Autodesk Inventor part; units mm, degrees
ref_plane "YZ Plane" through (0, 0, 0) normal (1, 0, 0) x (0, 1, 0)
ref_plane "XZ Plane" through (0, 0, 0) normal (0, 1, 0) x (-1, 0, 0)
ref_plane "XY Plane" through (0, 0, 0) normal (0, 0, 1) x (1, 0, 0)
sketch "Sombreado_1" plane through (0, 0, 0) normal (0, 0, 1) x (1, 0, 0)
  point P0 (0, 0)
sketch "Sombreado_2" plane through (0, 0, 0) normal (0, 0, 1) x (1, 0, 0)
  point P0 (0, 0)
sketch "Sombreado_3" plane through (0, 0, 0) normal (0, 0, 1) x (1, 0, 0)
  point P0 (0, 0)
sketch "Boceto1" plane through (0, 0, 0) normal (0, 1, 0) x (-1, 0, 0)
  line L0 (30.3882, 1.25) -> (30.8882, 1.25)
  line L1 (0, -6.75) -> (75, -6.75)
  line L2 (75, -6.75) -> (75, 18.25)
  line L3 (75, 18.25) -> (0, 18.25)
  line L4 (0, 18.25) -> (0, -6.75)
  arc A0 (21.3882, 1.25) -> (30.8882, 1.25) centre (26.1382, 1.25) ccw
  arc A1 (21.8882, 1.25) -> (30.3882, 1.25) centre (26.1382, 1.25) ccw
  line L5 (21.3882, 1.25) -> (21.8882, 1.25)
  line L6 (1.8, 2.5) -> (5.3, 2.5)
  line L7 (1.8, 2.5) -> (1.8, 3)
  line L8 (1.8, 3) -> (1, 3)
  line L9 (1, 3) -> (1, 2.5)
  line L10 (1, 0) -> (0, 0)
  line L11 (1, 0) -> (1, -0.5)
  line L12 (1, -0.5) -> (1.8, -0.5)
  line L13 (1.8, -0.5) -> (1.8, 0)
  line L14 (5.3, 0) -> (1.8, 0)
  line L15 (0, 2.5) -> (1, 2.5)
  line L16 (1.8, 11.5) -> (5.3, 11.5)
  line L17 (5.3, 9) -> (1.8, 9)
  line L18 (1, 9) -> (0, 9)
  line L19 (0, 11.5) -> (1, 11.5)
  line L20 (1.8, 11.5) -> (1.8, 12)
  line L21 (1.8, 12) -> (1, 12)
  line L22 (1, 12) -> (1, 11.5)
  line L23 (1, 9) -> (1, 8.5)
  line L24 (1, 8.5) -> (1.8, 8.5)
  line L25 (1.8, 8.5) -> (1.8, 9)
  line L26 (44.6082, 1.25) -> (44.1082, 1.25)
  arc A2 (44.1082, 1.25) -> (53.6082, 1.25) centre (48.8582, 1.25) ccw
  arc A3 (44.6082, 1.25) -> (53.1082, 1.25) centre (48.8582, 1.25) ccw
  line L27 (53.6082, 1.25) -> (53.1082, 1.25)
  line L28 (73.1964, 2.5) -> (69.6964, 2.5)
  line L29 (69.6964, 0) -> (73.1964, 0)
  line L30 (73.9964, 0) -> (74.9964, 0)
  line L31 (74.9964, 2.5) -> (73.9964, 2.5)
  line L32 (73.1964, 2.5) -> (73.1964, 3)
  line L33 (73.1964, 3) -> (73.9964, 3)
  line L34 (73.9964, 3) -> (73.9964, 2.5)
  line L35 (73.9964, 0) -> (73.9964, -0.5)
  line L36 (73.9964, -0.5) -> (73.1964, -0.5)
  line L37 (73.1964, -0.5) -> (73.1964, 0)
  line L38 (73.1964, 11.5) -> (69.6964, 11.5)
  line L39 (69.6964, 9) -> (73.1964, 9)
  line L40 (73.9964, 9) -> (74.9964, 9)
  line L41 (74.9964, 11.5) -> (73.9964, 11.5)
  line L42 (73.1964, 11.5) -> (73.1964, 12)
  line L43 (73.1964, 12) -> (73.9964, 12)
  line L44 (73.9964, 12) -> (73.9964, 11.5)
  line L45 (73.9964, 9) -> (73.9964, 8.5)
  line L46 (73.9964, 8.5) -> (73.1964, 8.5)
  line L47 (73.1964, 8.5) -> (73.1964, 9)
  line L48 (75, 18.25) -> (75, 43.25)
  line L49 (75, 43.25) -> (0, 43.25)
  line L50 (0, 43.25) -> (0, 18.25)
  line L51 (5.3, 11.5) -> (5.3, 9)
  line L52 (5.3, 2.5) -> (5.3, 0)
  line L53 (69.6964, 11.5) -> (69.6964, 9)
  line L54 (69.6964, 2.5) -> (69.6964, 0)
  circle A4 centre (26.1382, 1.25) radius 3.25
  circle A5 centre (48.8582, 1.25) radius 3.25
  circle A6 centre (26.1382, 26.25) radius 3.25
  circle A7 centre (48.8582, 26.25) radius 3.25
  line L55 (75, 43.25) -> (75, 68.25)
  line L56 (75, 68.25) -> (0, 68.25)
  line L57 (0, 68.25) -> (0, 43.25)
  circle A8 centre (26.1382, 51.25) radius 3.25
  circle A9 centre (48.8582, 51.25) radius 3.25
  point P0 (0, 0)
sketch "Boceto3" plane through (0, 0, 0) normal (0, 1, 0) x (-1, 0, 0)
  line L0 (0, 0) -> (-75, 0)
  line L1 (-75, 0) -> (-75, -25)
  line L2 (-75, -25) -> (0, -25)
  line L3 (0, -25) -> (0, 0)
  line L4 (0, 0) -> (-75, 0)
  line L5 (-75, 0) -> (-75, -25)
  line L6 (-75, -25) -> (0, -25)
  line L7 (0, -25) -> (0, 0)
  dimension "d4" = 75
  dimension "d5" = 25
  dimension "d6" = 75
  dimension "d7" = 25
extrude "Extrusión1" add sketch "Boceto3" along normal blind 2
sketch "Boceto4" plane through (0, 2, 0) normal (0, 1, 0) x (1, 0, 0)
  line L0 (-1.8065, 18.25) -> (1.0036, 18.25)
  line L1 (-1.8065, 15.75) -> (1.0036, 15.75)
  line L2 (1.0036, 15.75) -> (1.0036, 15.25)
  line L3 (1.8036, 15.75) -> (1.8036, 15.25)
  line L4 (1.0036, 18.75) -> (1.8036, 18.75)
  line L5 (1.0036, 15.25) -> (1.8036, 15.25)
  line L6 (1.0036, 18.25) -> (1.0036, 18.75)
  line L7 (1.8036, 18.75) -> (1.8036, 18.25)
  line L8 (1.8036, 18.25) -> (5.3036, 18.25)
  line L9 (1.8036, 15.75) -> (5.3036, 15.75)
  line L10 (5.3036, 18.25) -> (5.3036, 15.75)
  line L11 (-1.5403, 9.25) -> (-1.5403, 6.75)
  line L12 (-1.5403, 9.25) -> (1.0036, 9.25)
  line L13 (-1.5403, 6.75) -> (1.0036, 6.75)
  line L14 (1.0036, 6.75) -> (1.0036, 6.25)
  line L15 (1.8036, 6.75) -> (1.8036, 6.25)
  line L16 (1.0036, 9.75) -> (1.8036, 9.75)
  line L17 (1.0036, 6.25) -> (1.8036, 6.25)
  line L18 (1.0036, 9.25) -> (1.0036, 9.75)
  line L19 (1.8036, 9.75) -> (1.8036, 9.25)
  line L20 (1.8036, 9.25) -> (5.3036, 9.25)
  line L21 (1.8036, 6.75) -> (5.3036, 6.75)
  line L22 (5.3036, 9.25) -> (5.3036, 6.75)
  circle A0 centre (26.1418, 8) radius 3.25
  arc A1 (21.3918, 8) -> (30.8918, 8) centre (26.1418, 8) ccw
  arc A2 (21.8918, 8) -> (30.3918, 8) centre (26.1418, 8) ccw
  line L23 (30.3918, 8) -> (30.8918, 8)
  line L24 (21.8918, 8) -> (21.3918, 8)
  line L25 (-1.8065, 18.25) -> (-1.8065, 15.75)
  line L26 (5.3036, 15.75) -> (7.3036, 16.75)
  line L27 (5.3036, 18.25) -> (7.3036, 17.25)
  line L28 (7.3036, 16.75) -> (9.4436, 16.75)
  line L29 (9.4436, 16.75) -> (13.6836, 12.5)
  line L30 (9.7963, 17.1027) -> (9.7972, 17.1036)
  line L31 (14.1397, 12.749) -> (9.6494, 17.25)
  line L32 (7.3036, 17.25) -> (9.6494, 17.25)
  line L33 (5.3036, 9.25) -> (7.3036, 8.25)
  line L34 (5.3036, 6.75) -> (7.3036, 7.75)
  line L35 (7.3036, 8.25) -> (9.4436, 8.25)
  line L36 (9.4436, 8.25) -> (13.6836, 12.5)
  line L37 (14.1397, 12.251) -> (9.6494, 7.75)
  line L38 (7.3036, 7.75) -> (9.6494, 7.75)
  line L39 (14.1397, 12.749) -> (26.1418, 12.749)
  line L40 (14.1397, 12.251) -> (26.1418, 12.251)
  arc A3 (30.3918, 8) -> (26.1418, 12.25) centre (26.1418, 8) ccw
  arc A4 (30.8918, 8) -> (26.1418, 12.75) centre (26.1418, 8) ccw
  line L41 (0, 0) -> (75, 0)
  line L42 (75, 25) -> (0, 25)
  line L43 (76.8065, 18.25) -> (73.9964, 18.25)
  line L44 (76.8065, 15.75) -> (73.9964, 15.75)
  line L45 (73.9964, 15.75) -> (73.9964, 15.25)
  line L46 (73.1964, 15.75) -> (73.1964, 15.25)
  line L47 (73.9964, 18.75) -> (73.1964, 18.75)
  line L48 (73.9964, 15.25) -> (73.1964, 15.25)
  line L49 (73.9964, 18.25) -> (73.9964, 18.75)
  line L50 (73.1964, 18.75) -> (73.1964, 18.25)
  line L51 (73.1964, 18.25) -> (69.6964, 18.25)
  line L52 (73.1964, 15.75) -> (69.6964, 15.75)
  line L53 (69.6964, 18.25) -> (69.6964, 15.75)
  line L54 (69.6964, 9.25) -> (69.6964, 6.75)
  line L55 (73.1964, 6.75) -> (73.1964, 6.25)
  line L56 (73.1964, 6.75) -> (69.6964, 6.75)
  line L57 (73.1964, 9.75) -> (73.1964, 9.25)
  line L58 (73.9964, 6.75) -> (73.9964, 6.25)
  line L59 (73.9964, 6.25) -> (73.1964, 6.25)
  line L60 (73.9964, 9.75) -> (73.1964, 9.75)
  line L61 (73.9964, 9.25) -> (73.9964, 9.75)
  line L62 (76.5403, 9.25) -> (76.5403, 6.75)
  line L63 (76.5403, 9.25) -> (73.9964, 9.25)
  line L64 (76.5403, 6.75) -> (73.9964, 6.75)
  line L65 (73.1964, 9.25) -> (69.6964, 9.25)
  circle A5 centre (48.8582, 8) radius 3.25
  arc A6 (44.1082, 8) -> (53.6082, 8) centre (48.8582, 8) ccw
  arc A7 (44.6082, 8) -> (53.1082, 8) centre (48.8582, 8) ccw
  line L66 (44.6082, 8) -> (44.1082, 8)
  line L67 (53.1082, 8) -> (53.6082, 8)
  line L68 (76.8065, 18.25) -> (76.8065, 15.75)
  line L69 (69.6964, 15.75) -> (67.6964, 16.75)
  line L70 (69.6964, 18.25) -> (67.6964, 17.25)
  line L71 (67.6964, 16.75) -> (65.5564, 16.75)
  line L72 (65.5564, 16.75) -> (61.3164, 12.5)
  line L73 (65.2037, 17.1027) -> (65.2028, 17.1036)
  line L74 (60.8603, 12.749) -> (65.3506, 17.25)
  line L75 (67.6964, 17.25) -> (65.3506, 17.25)
  line L76 (67.6964, 8.25) -> (65.5564, 8.25)
  line L77 (67.6964, 7.75) -> (65.3506, 7.75)
  line L78 (60.8603, 12.251) -> (65.3506, 7.75)
  line L79 (65.5564, 8.25) -> (61.3164, 12.5)
  line L80 (69.6964, 9.25) -> (67.6964, 8.25)
  line L81 (69.6964, 6.75) -> (67.6964, 7.75)
  line L82 (60.8603, 12.749) -> (48.8582, 12.749)
  line L83 (60.8603, 12.251) -> (48.8582, 12.251)
  arc A8 (48.8582, 12.25) -> (44.6082, 8) centre (48.8582, 8) ccw
  arc A9 (48.8582, 12.75) -> (44.1082, 8) centre (48.8582, 8) ccw
extrude "Extrusión2" cut sketch "Boceto4" against normal blind 2 contours L0 L6 L4 L7 L8 L10 L9 L3 L5 L2 L1 L25 | A1 L24 A2 L23 | L22 L21 L15 L17 L14 L13 L11 L12 L18 L16 L19 L20 | A0 | L68 L44 L45 L48 L46 L52 L53 L51 L50 L47 L49 L43 | L66 A7 L67 A6 | L65 L57 L60 L61 L63 L62 L64 L58 L59 L55 L56 L54 | A5
sketch "Boceto5" plane through (0, 2, 0) normal (0, 1, 0) x (1, 0, 0)
  line L0 (5.3036, 18.25) -> (5.3036, 15.75)
  line L1 (5.3036, 9.25) -> (5.3036, 6.75)
  line L2 (5.3036, 15.75) -> (7.3036, 16.75)
  line L3 (5.3036, 18.25) -> (7.3036, 17.25)
  line L4 (7.3036, 16.75) -> (9.4436, 16.75)
  line L5 (9.4436, 16.75) -> (13.6836, 12.5)
  line L6 (9.7963, 17.1027) -> (9.7972, 17.1036)
  line L7 (14.1397, 12.749) -> (9.6494, 17.25)
  line L8 (7.3036, 17.25) -> (9.6494, 17.25)
  line L9 (7.3036, 8.25) -> (9.4436, 8.25)
  line L10 (7.3036, 7.75) -> (9.6494, 7.75)
  line L11 (14.1397, 12.251) -> (9.6494, 7.75)
  line L12 (9.4436, 8.25) -> (13.6836, 12.5)
  line L13 (5.3036, 9.25) -> (7.3036, 8.25)
  line L14 (5.3036, 6.75) -> (7.3036, 7.75)
  line L15 (14.1397, 12.749) -> (26.1418, 12.749)
  line L16 (14.1397, 12.251) -> (26.1418, 12.251)
  line L17 (30.8908, 8) -> (30.3928, 8)
  arc A0 (30.3928, 8) -> (26.1418, 12.251) centre (26.1418, 8) ccw
  arc A1 (30.8908, 8) -> (26.1418, 12.749) centre (26.1418, 8) ccw
  line L18 (69.6964, 18.25) -> (69.6964, 15.75)
  line L19 (69.6964, 9.25) -> (69.6964, 6.75)
  line L20 (69.6964, 15.75) -> (67.6964, 16.75)
  line L21 (69.6964, 18.25) -> (67.6964, 17.25)
  line L22 (67.6964, 16.75) -> (65.5564, 16.75)
  line L23 (65.5564, 16.75) -> (61.3164, 12.5)
  line L24 (65.2037, 17.1027) -> (65.2028, 17.1036)
  line L25 (60.8603, 12.749) -> (65.3506, 17.25)
  line L26 (67.6964, 17.25) -> (65.3506, 17.25)
  line L27 (67.6964, 8.25) -> (65.5564, 8.25)
  line L28 (67.6964, 7.75) -> (65.3506, 7.75)
  line L29 (60.8603, 12.251) -> (65.3506, 7.75)
  line L30 (65.5564, 8.25) -> (61.3164, 12.5)
  line L31 (69.6964, 9.25) -> (67.6964, 8.25)
  line L32 (69.6964, 6.75) -> (67.6964, 7.75)
  line L33 (60.8603, 12.749) -> (48.8582, 12.749)
  line L34 (60.8603, 12.251) -> (48.8582, 12.251)
  line L35 (44.1092, 8) -> (44.6072, 8)
  arc A2 (48.8582, 12.251) -> (44.6072, 8) centre (48.8582, 8) ccw
  arc A3 (48.8582, 12.749) -> (44.1092, 8) centre (48.8582, 8) ccw
  point P0 (0, 0)
extrude "Extrusión3" cut sketch "Boceto5" against normal blind 1
properties part number "2ureactor Torus" material "PPS Plastic"
Here's how the part is built. I have some questions about the finished solid (model axes, mm). A direction names the side the tool comes from. Round coordinates to 2 decimals unless told otherwise and drop trailing zeros. Loops run counter-clockwise (first coordinate to the right, second up) from the corner with the lowest first, then second, coordinate; pieces in that order, holes last. Notation, with made-up numbers: (31.5, 40) -> (59.5, 40) arc R14 cw to (59.5, 46) -> close; hole circle Ø7 at (58, -28.75). An arc over 180 degrees is marked (long way). Write each question's results on one line, items separated by ' | '.
(1) We'd pull the mould along Z, two halves only. Please class faces 5 (the face through (38, 2, -12)), 6 (the face through (38, 1, -25)), 7 (the face through (45.537, 1.507, -11.395)): released by +Z, released by -Z, zero draft, split by the parting line, or undercut.
Worked answers:
face 5: zero draft | face 6: released by -Z | face 7: undercut
(2) If we section it at D-D, the plane x = 25: List the corners of the cut face in (y, z) for me, then the cut area to 3 significant figures.
Worked answers:
outline: (0, -25) -> (2, -25) -> (2, -12.75) -> (1, -12.75) -> (1, -12.25) -> (2, -12.25) -> (2, -11.04) -> (0, -11.04) -> close; (0, -4.96) -> (2, -4.96) -> (2, -3.91) -> (0, -3.91) -> close; (0, -3.39) -> (2, -3.39) -> (2, 0) -> (0, 0) -> close | area: 36.3 mm2
(3) If I drill on L1, parallel to Z at x = 66.5, y = 1.25; L2, parallel to Z at x = 71.5, y = 0.1; L3, parallel to Z at x = 17.5, y = 1.15, over which ranges is the centre line in solid material (lowest first)?
Worked answers:
L1: -25 to -17.25, -16.75 to -8.25, -7.75 to 0 | L2: -25 to -18.25, -15.75 to -9.25, -6.75 to 0 | L3: -25 to -12.75, -12.25 to 0
(4) For faces 1 (the face through (11.926, 1.507, -10.032)), 2 (the face through (4, 1, -6.75)), 3 (the face through (71, 1, -18.25)), 4 (the face through (0, 1, -13)), which set-ups out of +Z, -Z, +X, -X, +Y, -Y let a thin tool reach every point of the face, with its end or its side?
Worked answers:
face 1: +Y | face 2: -X, +Y, -Y | face 3: +X, +Y, -Y | face 4: +Z, -Z, -X, +Y, -Y
(5) If we section it at B-B, the plane z = -10.5: List the corners of the cut face in (x, y) for me.
Worked answers:
outline: (0, 0) -> (24.07, 0) -> (24.07, 2) -> (12.39, 2) -> (12.39, 1) -> (11.69, 1) -> (11.69, 2) -> (0, 2) -> close; (28.22, 0) -> (46.78, 0) -> (46.78, 2) -> (45.42, 2) -> (45.42, 1) -> (44.82, 1) -> (44.82, 2) -> (30.18, 2) -> (30.18, 1) -> (29.58, 1) -> (29.58, 2) -> (28.22, 2) -> close; (50.93, 0) -> (75, 0) -> (75, 2) -> (63.31, 2) -> (63.31, 1) -> (62.61, 1) -> (62.61, 2) -> (50.93, 2) -> close
(6) For P1, Ø0.6, axis at x = 73.5, y = 1.5, coming from the +Z side; P2, Ø0.8, axis at y = 0.5, z = -16.5, coming from the +X side, each with a flat end and sliding along its axis, tell me the tip position at first contact or that it passes through.
Worked answers:
P1: z = 0 | P2: x = 69.7
(7) If we section it at A-A, the plane x = 51: List the corners of the cut face in (y, z) for me, then the cut area to 3 significant figures.
Worked answers:
outline: (0, -25) -> (2, -25) -> (2, -12.75) -> (1, -12.75) -> (1, -12.25) -> (2, -12.25) -> (2, -10.44) -> (0, -10.44) -> close; (0, -5.56) -> (2, -5.56) -> (2, -4.33) -> (0, -4.33) -> close; (0, -3.76) -> (2, -3.76) -> (2, 0) -> (0, 0) -> close | area: 38.6 mm2
(8) If we section it at C-C, the plane x = 64: List the corners of the cut face in (y, z) for me, then the cut area to 3 significant figures.
Worked answers:
outline: (0, -25) -> (2, -25) -> (2, -15.9) -> (1, -15.9) -> (1, -15.19) -> (2, -15.19) -> (2, -9.81) -> (1, -9.81) -> (1, -9.1) -> (2, -9.1) -> (2, 0) -> (0, 0) -> close | area: 48.6 mm2
